Model file for the job. Use its own axes, mm. Round coordinates to 2 decimals unless told otherwise and drop trailing zeros. Order: outer loops, then holes, each group sorted by start corner. A loop starts at its lowest first (then second) coordinate and runs counter-clockwise, first axis right, second up. Notation, with made-up numbers: (-2.5, 57.5) - (42.5, 57.5) arc R16 cw to (42.5, 83.5) - close; hole circle Ø8 at (46.25, 72.25). An arc over 180 degrees is marked (long way). Answer as CSV lines item,"result". Start each with the question number.
1. Band-saw the part on B-B on y = 2. List the corners of the cut face in (x, z) (3 decimals), then the cut area to 3 significant figures.
2. Band-saw the part on C-C on z = 7.5. List the corners of the cut face in (x, y) (3 decimals), then the cut area to 3 significant figures.
3. Pull direction Z, two halves, no side cores. Call faces 1 (the face through (100, 3.175, 0)), 2 (the face through (220.44, 1.57, -17.14)), 3 (the face through (53.83, 1.57, -0.95)): released by +Z, released by -Z, zero draft, split by the parting line, or undercut.
4. Wall check: line 1 along X through (y, z) = (1.5, 0) (3 decimals); line 2 along X through (y, z) = (1.65, 8); line 3 along X through (y, z) = (2, -1). Give the ranges that are in metal, low to high. Write a range as [from, to].
5. Band-saw the part on D-D on x = 50.8. List the corners of the cut face in (y, z) (3 decimals).
6. Band-saw the part on A-A on x = 0. List the corners of the cut face in (y, z) (3 decimals).
```python
from build123d import *

# Parameters (mm, degrees)
SKETCH1_R           = 12.7
SKETCH1_R_2         = 3.175
BOSS_EXTRUDE1_DEPTH = 3.175


with BuildPart() as part:
    # Sketch1 → Boss-Extrude1 (new body)
    with BuildSketch(Plane(origin=(0, 0, 0), x_dir=(1, 0, 0), z_dir=(0, 1, 0))):
        with BuildLine():
            Line((-12.7, -19.05), (215.9, -19.05))
            ThreePointArc((215.9, -19.05), (220.390128061, -17.190128061), (222.25, -12.7))
            Line((222.25, -12.7), (222.25, 12.7))
            ThreePointArc((222.25, 12.7), (220.390128061, 17.190128061), (215.9, 19.05))
            Line((215.9, 19.05), (-12.7, 19.05))
            ThreePointArc((-12.7, 19.05), (-17.190128061, 17.190128061), (-19.05, 12.7))
            Line((-19.05, 12.7), (-19.05, -12.7))
            ThreePointArc((-19.05, -12.7), (-17.190128061, -17.190128061), (-12.7, -19.05))
        make_face()
        Circle(SKETCH1_R, mode=Mode.SUBTRACT)
        with Locations((203.2, 0)):
            Circle(SKETCH1_R, mode=Mode.SUBTRACT)
        with Locations((50.8, 0)):
            Circle(SKETCH1_R_2, mode=Mode.SUBTRACT)
        with Locations((152.4, 0)):
            Circle(SKETCH1_R_2, mode=Mode.SUBTRACT)
    extrude(amount=BOSS_EXTRUDE1_DEPTH)


solid = part.part
```
Reply:
1,outline,"(-19.05, -12.7) arc R6.35 ccw to (-12.7, -19.05) - (215.9, -19.05) arc R6.35 ccw to (222.25, -12.7) - (222.25, 12.7) arc R6.35 ccw to (215.9, 19.05) - (-12.7, 19.05) arc R6.35 ccw to (-19.05, 12.7) - close; hole circle Ø25.4 at (0, 0); hole circle Ø6.35 at (50.8, 0); hole circle Ø6.35 at (152.4, 0); hole circle Ø25.4 at (203.2, 0)"
1,area,"8,080 mm2"
2,outline,"(-19.05, 0) - (-10.249, 0) - (-10.249, 3.175) - (-19.05, 3.175) - close; (10.249, 0) - (192.951, 0) - (192.951, 3.175) - (10.249, 3.175) - close; (213.449, 0) - (222.25, 0) - (222.25, 3.175) - (213.449, 3.175) - close"
2,area,"636 mm2"
3,face 1,"zero draft"
3,face 2,"released by -Z"
3,face 3,"undercut"
4,line 1,"x = [-19.05, -12.7], [12.7, 47.625], [53.975, 149.225], [155.575, 190.5], [215.9, 222.25]"
4,line 2,"x = [-19.05, -9.86], [9.86, 193.34], [213.06, 222.25]"
4,line 3,"x = [-19.05, -12.66], [12.66, 47.79], [53.81, 149.39], [155.41, 190.54], [215.86, 222.25]"
5,outline,"(0, -19.05) - (3.175, -19.05) - (3.175, -3.175) - (0, -3.175) - close; (0, 3.175) - (3.175, 3.175) - (3.175, 19.05) - (0, 19.05) - close"
6,outline,"(0, -19.05) - (3.175, -19.05) - (3.175, -12.7) - (0, -12.7) - close; (0, 12.7) - (3.175, 12.7) - (3.175, 19.05) - (0, 19.05) - close"
